```python
from build123d import *

# Parameters (mm, degrees)
F0_R     = 5
F1_DEPTH = 5
F2_R     = 3
F3_R     = 6
F3_R_2   = 5
F4_DEPTH = 2
F5_R     = 0.99999
F6_R     = 1.75
F7_DEPTH = 4


# Not quite as in the source:
# - a fillet or chamfer is up to 0.001 mm smaller than in the source, because OpenCascade refuses the exact size


with BuildPart() as f1:
    # F0 (on Top) → F1 (new body)
    with BuildSketch(Plane.XY):
        Circle(F0_R)
    extrude(amount=F1_DEPTH)

    # F2
    f2_edges = [f1.edges().sort_by_distance(p)[0] for p in [
        (-5, 0, 5),
    ]]
    fillet(f2_edges, radius=F2_R)

    # F3 (on face) → F4 (join)
    with BuildSketch(Plane(origin=(0, 0, 0), x_dir=(1, 0, 0), z_dir=(0, 0, -1))):
        Circle(F3_R)
        Circle(F3_R_2, mode=Mode.SUBTRACT)
        Circle(F3_R_2)
    extrude(amount=F4_DEPTH)

    # F5 (radius 1 in the source; OpenCascade refuses exactly that, so slightly less here)
    f5_edges = [f1.edges().sort_by_distance(p)[0] for p in [
        (-6, 0, 0),
    ]]
    fillet(f5_edges, radius=F5_R)

    # F6 (on face) → F7 (cut)
    with BuildSketch(Plane(origin=(0, 0, -2), x_dir=(1, 0, 0), z_dir=(0, 0, -1))):
        Circle(F6_R)
    extrude(amount=-F7_DEPTH, mode=Mode.SUBTRACT)


solid = f1.part
```
Design review of the part built by this model. Coordinates are the model's own, in mm. A direction names the side the tool comes from. Give positions to 0.01 mm unless a question says otherwise; leave off trailing zeros. Write each loop counter-clockwise with the first axis right and the second up, starting at its lowest first coordinate (ties: lowest second). Pieces come first, ordered by that corner, then holes. Notation, with made-up numbers: (-8.5, 89) - (29.5, 89) arc R18 cw to (29.5, 102) - close; hole circle Ø3 at (53.25, 88). An arc over 180 degrees is marked (long way). Return JSON: item names as keys, results as strings. Group by question number.
(1) We need section A-A, the plane z = 0.25. Give the boundary of the cut face in (x, y), then the cut area to 3 significant figures.
(2) Insertion check: pin 1 (2 mm diameter, centred on x = 4, z = 4, fed in from -Y); pin 2 (1.8 mm diameter, centred on x = 0, y = 0.5, fed in from -Z); pin 3 (3 mm diameter, centred on y = 1.5, z = 3.5, fed in from +X); pin 4 (4 mm diameter, centred on x = -1, y = 1, fed in from -Z). Each pin has a flat end and moves straight along its axis. Give the tip position at first contact, or say it passes through.
(3) Machinability: for faces 4 (the flat face through (0, 0, 5)), 5 (the flat face through (0, 0, 2)), which of the approach directions +Z, -Z, +X, -X, +Y, -Y give a long, thin tool a straight path to every point of the face, cutting with its end or side? Answer none if there is none.
(4) To check wall thickness, follow probe 1 along Y at (x, z) = (0, 0.2); probe 2 along Z at (x, y) = (1.25, 1.75); probe 3 along X at (y, z) = (0, -0.5). State the ranges of each line that lie inside material, in increasing order.
(5) Mouldability with a two-part tool opening along Y and no side actions: class faces 1 (the flat face through (-1.4, -1.4, -2)), 2 (the cylindrical face through (-1.08, -4.88, 0.99)), 3 (the cylindrical face through (1.617, 0.67, -0.028)) as +Y half, -Y half, draft (parallel to the pull), parting line (faces both ways), or undercut.
Reported:
{
 "1": {"outline": "circle Ø10 at (0, 0); hole circle Ø3.5 at (0, 0)", "area": "68.9 mm2"},
 "2": {"pin 1": "stops at y = -3.38", "pin 2": "stops at z = 2", "pin 3": "stops at x = 4.95", "pin 4": "stops at z = -2"},
 "3": {"face 4": "+Z, +X, -X, +Y, -Y", "face 5": "-Z"},
 "4": {"probe 1": "y = -5 to -1.75, 1.75 to 5", "probe 2": "z = -2 to 5", "probe 3": "x = -5.87 to -1.75, 1.75 to 5.87"},
 "5": {"face 1": "draft", "face 2": "parting line", "face 3": "undercut"}
}
